from build123d import *

# Parameters (mm, degrees)
F0_R     = 20
F1_DEPTH = 50
F0_R_2   = 25
F2_DEPTH = 25
F3_SIZE  = 2.5
F4_SIZE  = 1.5


with BuildPart() as f1:
    # F0 (on Front) → F1 (new body)
    with BuildSketch(Plane.XZ):
        Circle(F0_R)
    extrude(amount=F1_DEPTH)

    # F0 (on Front) → F2 (join)
    with BuildSketch(Plane.XZ):
        Circle(F0_R_2)
        Circle(F0_R, mode=Mode.SUBTRACT)
    extrude(amount=F2_DEPTH)

    # F3
    f3_edges = [f1.edges().sort_by_distance(p)[0] for p in [
        (-20, -50, 0),
    ]]
    chamfer(f3_edges, length=F3_SIZE)

    # F4
    f4_edges = [f1.edges().sort_by_distance(p)[0] for p in [
        (-25, -25, 0),
    ]]
    chamfer(f4_edges, length=F4_SIZE)


solid = f1.part
CAD build for the part. Positions are in the model's coordinates, mm. A direction names the side the tool comes from. Round coordinates to 2 decimals unless told otherwise and drop trailing zeros. Loops run counter-clockwise (first coordinate to the right, second up) from the corner with the lowest first, then second, coordinate; pieces in that order, holes last.
(1) Cut at D-D (y = -40). Give the cut face in (x, z).
(2) Cut at C-C (y = -8). Give the cut face in (x, z).
(3) Drop flat-ended pins along their axis: pin 1 (1.5 mm diameter, centred on y = -30.5, z = 7, fed in from -X); pin 2 (3 mm diameter, centred on x = -5.5, y = -14, fed in from -Z); pin 3 (12 mm diameter, centred on x = 12, y = -17.5, fed in from +Z). Give the stop position or say it passes through.
(4) Cut at B-B (x = 0). Give the cut face in (y, z).
(5) Which spindle directions (+Z, -Z, +X, -X, +Y, -Y) get a long thin tool onto all of the face, cutting with end or side? Do faces 1 (the flat face through (0, 0, 0)), 2 (the flat face through (7, -25, 19)). Say none if no direction does.
(6) Cut at A-A (z = 0). Give the cut face in (x, y).
(7) Wall check: line 1 along Y through (x, z) = (5, -22); line 2 along Y through (x, z) = (-13.5, -14); line 3 along X through (y, z) = (-18, 4). Give the ranges that are in metal, low to high.
Findings below:
1. outline: circle Ø40 at (0, 0)
2. outline: circle Ø50 at (0, 0)
3. pin 1: stops at x = -19
3. pin 2: stops at z = -24.68
3. pin 3: stops at z = 24.27
4. outline: (-50, -17.5) - (-47.5, -20) - (-25, -20) - (-25, -23.5) - (-23.5, -25) - (0, -25) - (0, 25) - (-23.5, 25) - (-25, 23.5) - (-25, 20) - (-47.5, 20) - (-50, 17.5) - close
5. face 1: +Z, -Z, +X, -X, +Y
5. face 2: -Y
6. outline: (-25, -23.5) - (-23.5, -25) - (-20, -25) - (-20, -47.5) - (-17.5, -50) - (17.5, -50) - (20, -47.5) - (20, -25) - (23.5, -25) - (25, -23.5) - (25, 0) - (-25, 0) - close
7. line 1: y = -25 to 0
7. line 2: y = -48.05 to 0
7. line 3: x = -24.68 to 24.68
